from build123d import *

# Parameters (mm, degrees)
F3_SIZE = 2
F4_SIZE = 0.5


# Not quite as in the source:
# - a fillet or chamfer that OpenCascade refuses, or shapes differently, is made with other operations: its cross-section is extruded or revolved along the edge and cut away or added


with BuildPart() as f1:
    # F0 (on Front) → F1 (revolve)
    with BuildSketch(Plane.XZ):
        Polygon((0, 24.5), (0, 0), (19, 0), (19, 9.5), (93, 9.5), (93, 12), (78, 12), (78, 17.5), (18, 17.5), (18, 15), (10, 15), (10, 24.5), align=None)
    revolve(axis=Axis((9.5, 0, 0), (-1, 0, 0)))

    # F2: fillet of radius 4.15 on 2 edges, made by hand

    # F2_s1 → F2_t2 (revolve)
    with BuildSketch(Plane.XZ):
        with BuildLine():
            ThreePointArc((14.15, 15), (11.2155068581, 16.2155068581), (10, 19.15))
            Line((10, 19.15), (10, 15))
            Line((10, 15), (14.15, 15))
        make_face()
    revolve(axis=Axis((10, 0, 0), (-1, 0, 0)))

    # F2_s3 → F2_t4 (revolve)
    with BuildSketch(Plane.XZ):
        with BuildLine():
            ThreePointArc((18, 17.5), (16.4697218419, 15.6808502483), (14.1921134471, 15))
            Line((14.1921134471, 15), (18, 15))
            Line((18, 15), (18, 17.5))
        make_face()
    revolve(axis=Axis((18, 0, 0), (-1, 0, 0)))

    # F3
    f3_edges = [f1.edges().sort_by_distance(p)[0] for p in [
        (0, 0, -24.5),
        (10, 0, -24.5),
    ]]
    chamfer(f3_edges, length=F3_SIZE)

    # F4
    f4_edges = [f1.edges().sort_by_distance(p)[0] for p in [
        (93, 0, -12),
        (93, 0, -9.5),
    ]]
    chamfer(f4_edges, length=F4_SIZE)


solid = f1.part
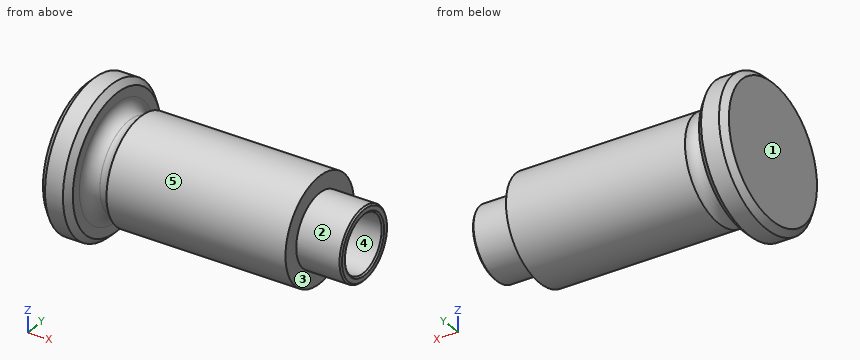
The listing builds one solid part. Answer for the finished solid, in the listing's coordinates (mm). Face numbers are marked on the shaded views. A direction names the side the tool comes from. Coordinates: 2 decimals unless noted, no trailing zeros. Loops run counter-clockwise (first coordinate to the right, second up) from the corner with the lowest first, then second, coordinate; pieces in that order, holes last. Notation, with made-up numbers: M 15,-20.5 L 66,-20.5 A35 ccw 66,13.5 Z; hole C -15.75,68 d2. An arc over 180 degrees is marked long. Answer in a Markdown table with one row per item.
1) Which of the six approach directions +Z, -Z, +X, -X, +Y, -Y give full straight-line access (tool end or side, diameter ignored) to the marked faces 1 and 2?
Answers below:
| item | result |
|---|---|
| face 1 | +Z, -Z, -X, +Y, -Y |
| face 2 | +X |
2) Determine the mould class of the marked faces 3, 4 and 5 for opening direction Y: released by +Y, released by -Y, zero draft, split by the parting line, or undercut.
Answers below:
| item | result |
|---|---|
| face 3 | zero draft |
| face 4 | undercut |
| face 5 | split by the parting line |
3) Find section C-C (x = 27). Determine the outline of the cut face in (y, z).
Answers below:
| item | result |
|---|---|
| outline | C 0,0 d35; hole C 0,0 d19 |
4) Find the intervals of material crossed by probe 1 along Y at (x, z) = (55, 0); probe 2 along X at (y, z) = (9, -17); probe 3 along X at (y, z) = (2, 9), in increasing order.
Answers below:
| item | result |
|---|---|
| probe 1 | -17.5 to -9.5, 9.5 to 17.5 |
| probe 2 | 0 to 10 |
| probe 3 | 0 to 19 |
5) Given pin 1 (3 mm diameter, centred on x = 49.5, y = -10.5, fed in from +Z); pin 2 (1.5 mm diameter, centred on x = 57.5, z = 3, fed in from +Y); pin 3 (5.5 mm diameter, centred on y = -3.5, z = 3, fed in from +X), each flat-ended and moving along its own axis, determine where each tip first touches the part or whether it passes through.
Answers below:
| item | result |
|---|---|
| pin 1 | z = 15.01 |
| pin 2 | y = 17.35 |
| pin 3 | x = 19 |
